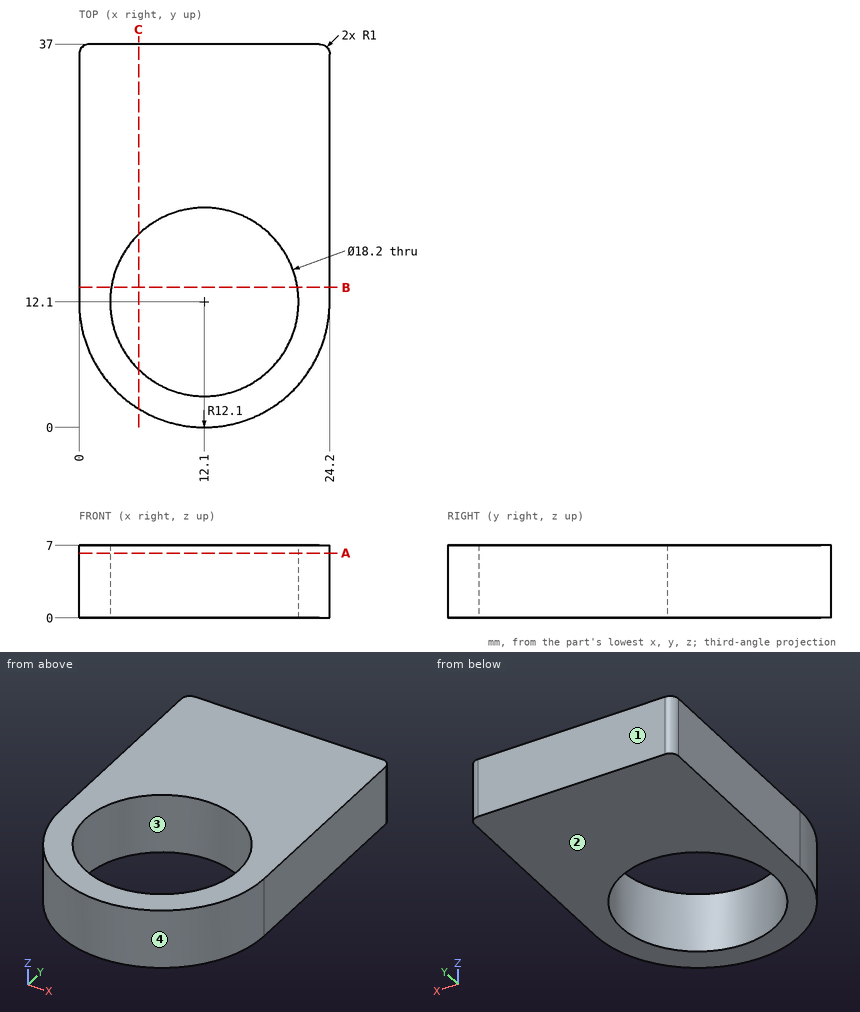
Geometry: see drawing. Coordinates: mm, zero at the bounding-box minimum. Coordinates: 2 decimals unless noted, no trailing zeros. Loops run counter-clockwise (first coordinate to the right, second up) from the corner with the lowest first, then second, coordinate; pieces in that order, holes last. Notation, with made-up numbers: M 32,-31 L 45,-31 A11 cw 45,-18 Z; hole C 44.25,8.5 d6. An arc over 180 degrees is marked long. Answer in a Markdown table with one row per item.
Q1. First-contact query: pin 1 (2 mm diameter, centred on y = 8.5, z = 1, fed in from -X); pin 2 (1.5 mm diameter, centred on x = 4.5, z = 3, fed in from -Y); pin 3 (4 mm diameter, centred on x = 16, z = 4.5, fed in from -Y). Flat tips, straight axial feed; report the tip coordinate or a pass-through.
Answers below:
| item | result |
|---|---|
| pin 1 | stops at x = 0.28 |
| pin 2 | stops at y = 2.13 |
| pin 3 | stops at y = 0.15 |
Q2. Section A-A on z = 6.25. Return the cut outline in (x, y), plus the area to 3 significant figures.
Answers below:
| item | result |
|---|---|
| outline | M 0,12.1 A12.1 ccw 24.2,12.1 L 24.2,36 A1 ccw 23.2,37 L 1,37 A1 ccw 0,36 Z; hole C 12.1,12.1 d18.2 |
| area | 572 mm^2 |
Q3. Ray query, probe 1 along Y at (x, z) = (12.1, 1.5); probe 2 along Y at (x, z) = (18, 2); probe 3 along X at (y, z) = (8.5, 6). Return the intervals inside material, ascending. Write a range as from..to.
Answers below:
| item | result |
|---|---|
| probe 1 | y = 0..3, 21.2..37 |
| probe 2 | y = 1.54..5.17, 19.03..37 |
| probe 3 | x = 0.55..3.74, 20.46..23.65 |
Q4. Draft query along Y for the marked faces 1, 2, 3 and 4. Return one class per face: pulls with the +Y half, pulls with the -Y half, needs draft (parallel to the pull), parting line crosses it, or undercut.
Answers below:
| item | result |
|---|---|
| face 1 | pulls with the +Y half |
| face 2 | needs draft |
| face 3 | undercut |
| face 4 | pulls with the -Y half |
Q5. Section B-B on y = 13.5. Return the cut outline in (x, z), plus the area to 3 significant figures.
Answers below:
| item | result |
|---|---|
| outline | M 0,0 L 3.11,0 L 3.11,7 L 0,7 Z; M 21.09,0 L 24.2,0 L 24.2,7 L 21.09,7 Z |
| area | 43.5 mm^2 |
Q6. Section C-C on x = 5.75. Return the cut outline in (y, z).
Answers below:
| item | result |
|---|---|
| outline | M 1.8,0 L 5.58,0 L 5.58,7 L 1.8,7 Z; M 18.62,0 L 37,0 L 37,7 L 18.62,7 Z |
